Input: dimensioned drawing with shaded views. Units: mm. Origin: part minimum x, y, z. A direction names the side the tool comes from. Give positions to 0.01 mm unless a question says otherwise; leave off trailing zeros. Write each loop counter-clockwise with the first axis right and the second up, starting at its lowest first coordinate (ties: lowest second). Pieces come first, ordered by that corner, then holes.
Q1. Pin query (flat end, axial travel): pin 1 Ø1.5 at (x, y) = (3, 7) entering from +Z; pin 2 Ø1.5 at (x, z) = (2.5, 3.5) entering from +Y; pin 3 Ø4 at (x, y) = (5.5, 2) entering from +Z; pin 4 Ø5.5 at (x, y) = (5, 5) entering from -Z. Return the tip coordinate at first contact, or that it passes through.
Q2. Section B-B (z = 3). Return the cut outline in (x, y), plus the area to 3 significant figures.
Q3. Mould query, pull axis X, two halves, no side actions, for the marked faces 1, 2, 3 and 4. Classes: +X half, -X half, draft (parallel to the pull), parting line (faces both ways), or undercut.
Q4. Section A-A (x = 7.25). Return the cut outline in (y, z).
Q5. Reachability of the marked faces 5, 6 and 7 from +Z, -Z, +X, -X, +Y, -Y: full face, straight path, thin tool, end or side. Return the list, or none.
Q6. Section C-C (y = 2.25). Return the cut outline in (x, z) (3 decimals), plus the area to 3 significant figures.
Q7. Section D-D (y = 7.5). Return the cut outline in (x, z).
Q8. Line query: line 1 (X direction, y = 5, z = 1.15); line 2 (Y direction, x = 5, z = 1.65); line 3 (Z direction, x = 2, y = 3.25). Output: solid intervals per line, ascending.
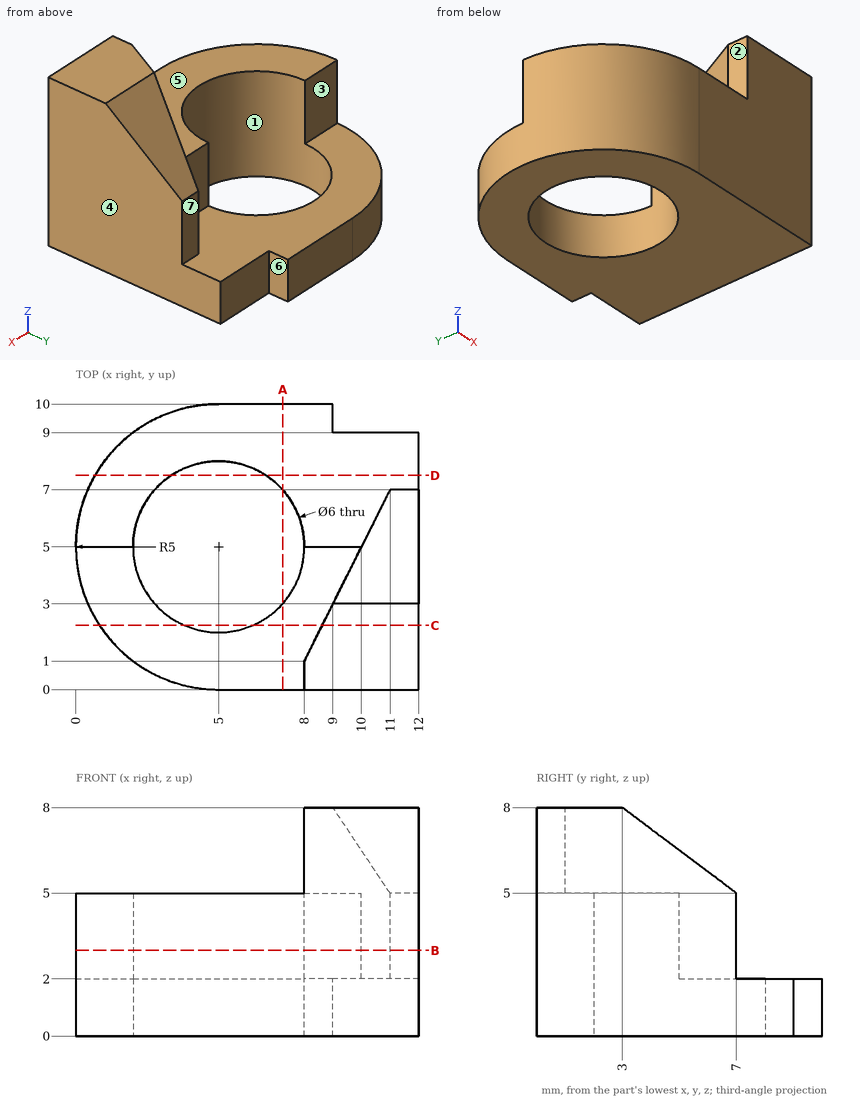
Computed:
1. pin 1: stops at z = 2
1. pin 2: stops at y = 5
1. pin 3: stops at z = 5
1. pin 4: passes through
2. outline: (0, 5) arc R5 ccw to (5, 0) - (12, 0) - (12, 7) - (11, 7) - (10, 5) - (8, 5) arc R3 cw to (2, 5) - close
2. area: 43.5 mm2
3. face 1: undercut
3. face 2: -X half
3. face 3: draft
3. face 4: +X half
4. outline: (0, 0) - (3.02, 0) - (3.02, 5) - (0, 5) - close; (6.98, 0) - (10, 0) - (10, 2) - (6.98, 2) - close
5. face 5: +Z, -X, +Y
5. face 6: +Z, -Z, +X, +Y
5. face 7: +Z, +X, -X, +Y
6. outline: (0.824, 0) - (3.801, 0) - (3.801, 5) - (0.824, 5) - close; (6.199, 0) - (12, 0) - (12, 8) - (8.625, 8) - (8.625, 5) - (6.199, 5) - close
6. area: 54.0 mm2
7. outline: (0.67, 0) - (3.34, 0) - (3.34, 2) - (0.67, 2) - close; (6.66, 0) - (12, 0) - (12, 2) - (6.66, 2) - close
8. line 1: x = 0 to 2, 8 to 12
8. line 2: y = 0 to 2, 8 to 10
8. line 3: z = 0 to 5
